Geometry check sheet. Reference: drawing and pictorial views, mm from the part's lowest x, y, z. A direction names the side the tool comes from. Give positions to 0.01 mm unless a question says otherwise; leave off trailing zeros. Order: outer loops, then holes, each group sorted by start corner. A loop starts at its lowest first (then second) coordinate and runs counter-clockwise, first axis right, second up. Notation, with made-up numbers: M 30,73 L 86,73 A4 cw 86,78 Z; hole C 61,-26.75 d9. An arc over 180 degrees is marked long. Use CSV: the item, a comma, the result in double quotes. Start each with the question number.
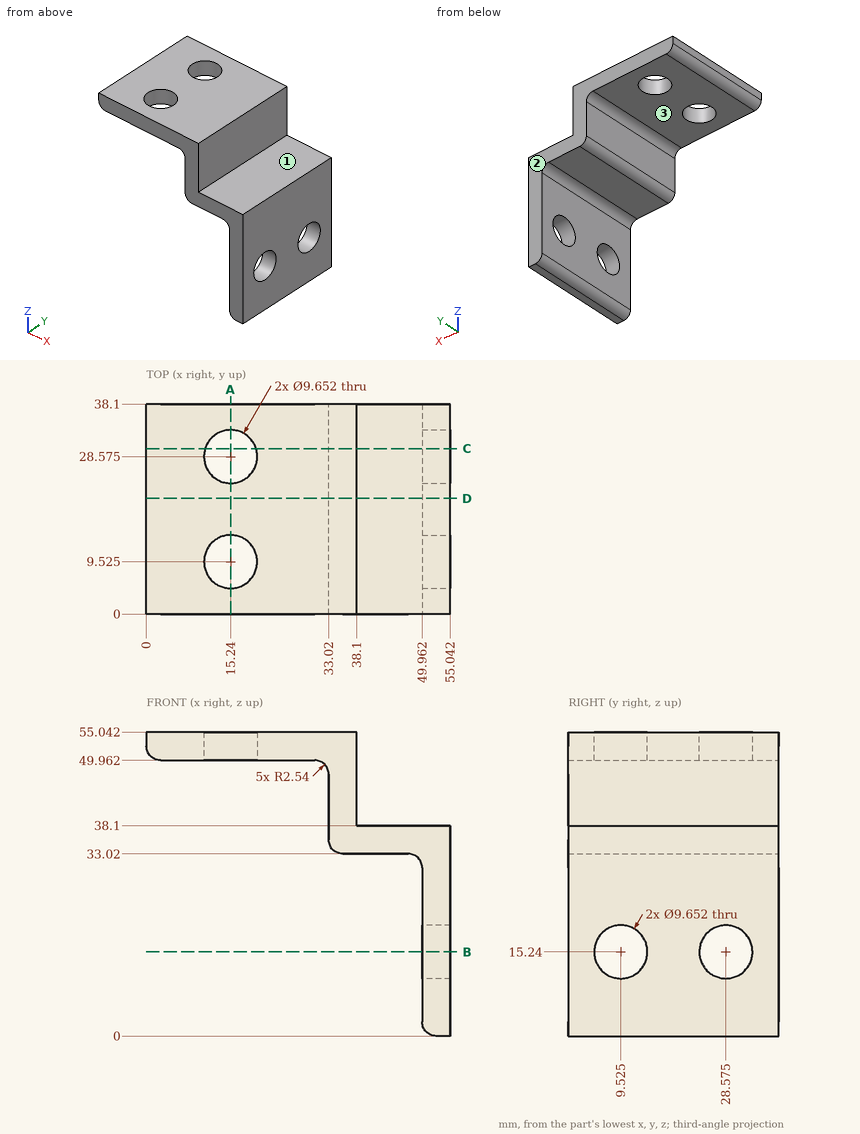
(1) Sectioned sample at C-C on y = 30. Record the cut outline in (x, z), then the cut area to 3 significant figures.
(2) Sectioned sample at D-D on y = 21. Record the cut outline in (x, z).
(3) Access from +Z, -Z, +X, -X, +Y, -Y to the whole of each face (thin tool, end or side, straight path). Record for the marked faces 1, 2 and 3.
(4) Thickness scan on line 1 (Y direction, x = 51, z = 15) (3 decimals); line 2 (Z direction, x = 43.5, y = 18.5); line 3 (Z direction, x = 24.5, y = 9). Record the ranges inside material, lowest first.
(5) Go/stop test with flat-tipped pins: P1, Ø11, axis at y = 28.575, z = 15.24, coming from the -X side; P2, Ø9.5, axis at y = 13.5, z = 43.5, coming from the -X side; P3, Ø12.5, axis at x = 15.24, y = 9.525, coming from the -Z side. Record where each tip stops, or that it passes through.
(6) Sectioned sample at B-B on z = 15.24. Record the cut outline in (x, y).
(7) Sectioned sample at A-A on x = 15.24. Record the cut outline in (y, z).
Responses:
1,outline,"M 0,52.5 A2.54 ccw 2.54,49.96 L 10.63,49.96 L 10.63,55.04 L 0,55.04 Z; M 19.85,49.96 L 30.48,49.96 A2.54 cw 33.02,47.42 L 33.02,35.56 A2.54 ccw 35.56,33.02 L 47.42,33.02 A2.54 cw 49.96,30.48 L 49.96,19.85 L 55.04,19.85 L 55.04,38.1 L 38.1,38.1 L 38.1,55.04 L 19.85,55.04 Z; M 49.96,2.54 A2.54 ccw 52.5,0 L 55.04,0 L 55.04,10.63 L 49.96,10.63 Z"
1,area,"438 mm2"
2,outline,"M 0,52.5 A2.54 ccw 2.54,49.96 L 30.48,49.96 A2.54 cw 33.02,47.42 L 33.02,35.56 A2.54 ccw 35.56,33.02 L 47.42,33.02 A2.54 cw 49.96,30.48 L 49.96,2.54 A2.54 ccw 52.5,0 L 55.04,0 L 55.04,38.1 L 38.1,38.1 L 38.1,55.04 L 0,55.04 Z"
3,face 1,"+Z, +X, +Y, -Y"
3,face 2,"+Z, -Z, +X, -X, +Y"
3,face 3,"-Z, -X, +Y, -Y"
4,line 1,"0 to 4.705, 14.345 to 23.755, 33.395 to 38.1"
4,line 2,"33.02 to 38.1"
4,line 3,"49.96 to 55.04"
5,P1,"x = 49.96"
5,P2,"x = 32.88"
5,P3,"z = 49.96"
6,outline,"M 49.96,0 L 55.04,0 L 55.04,4.7 L 49.96,4.7 Z; M 49.96,14.35 L 55.04,14.35 L 55.04,23.75 L 49.96,23.75 Z; M 49.96,33.4 L 55.04,33.4 L 55.04,38.1 L 49.96,38.1 Z"
7,outline,"M 0,49.96 L 4.7,49.96 L 4.7,55.04 L 0,55.04 Z; M 14.35,49.96 L 23.75,49.96 L 23.75,55.04 L 14.35,55.04 Z; M 33.4,49.96 L 38.1,49.96 L 38.1,55.04 L 33.4,55.04 Z"
